from build123d import *

# Parameters (mm, degrees)
SKETCH1_R           = 2.36
SKETCH1_R_2         = 1.625
BOSS_EXTRUDE1_DEPTH = 4.7625


with BuildPart() as part:
    # Sketch1 → Boss-Extrude1 (new body)
    with BuildSketch(Plane(origin=(0, 0, 0), x_dir=(1, 0, 0), z_dir=(0, 1, 0))):
        with BuildLine():
            Line((0, 6.35), (0, 11.65))
            Line((0, 11.65), (-12, 11.65))
            ThreePointArc((-12, 11.65), (-13.212057455, 11.518461446), (-14.367678703, 11.129970522))
            Line((-14.367678703, 11.129970522), (-27.367678703, 5.129970522))
            ThreePointArc((-27.367678703, 5.129970522), (-30.65, 0), (-27.367678703, -5.129970522))
            Line((-27.367678703, -5.129970522), (-14.367678703, -11.129970522))
            ThreePointArc((-14.367678703, -11.129970522), (-8.954912536, -10.759195555), (-6.35, -6))
            Line((-6.35, -6), (-6.35, 0))
            ThreePointArc((-6.35, 0), (-4.490128061, 4.490128061), (0, 6.35))
        make_face()
        with Locations((-25, 0)):
            Circle(SKETCH1_R, mode=Mode.SUBTRACT)
        with Locations((-12, 6)):
            Circle(SKETCH1_R_2, mode=Mode.SUBTRACT)
        with Locations((-12, -6)):
            Circle(SKETCH1_R_2, mode=Mode.SUBTRACT)
    boss_extrude1 = extrude(amount=BOSS_EXTRUDE1_DEPTH)

    # Mirror1: Boss-Extrude1 across plane
    add(boss_extrude1.mirror(Plane(origin=(0, 4.7625, -6.35), x_dir=(0, 0, 1), z_dir=(-1, 0, 0))))


solid = part.part
Can you work these out from the model? Positions are in its coordinate system, mm. Give positions to 0.01 mm unless a question says otherwise; leave off trailing zeros. Order: outer loops, then holes, each group sorted by start corner. A loop starts at its lowest first (then second) coordinate and runs counter-clockwise, first axis right, second up. Notation, with made-up numbers: M 55.5,55 L 98.5,55 A30 ccw 98.5,80 Z; hole C 12.5,12 d11. An arc over 180 degrees is marked long. One line per question, with ' | ' between items.
Item 1: Suppose I cut it at C-C, the plane x = 11. Write out the boundary of the cut face in (y, z).
Answer block:
outline: M 0,-11.65 L 4.76,-11.65 L 4.76,-7.28 L 0,-7.28 Z; M 0,-4.72 L 4.76,-4.72 L 4.76,4.72 L 0,4.72 Z; M 0,7.28 L 4.76,7.28 L 4.76,11.56 L 0,11.56 Z
Item 2: I'm going to push flat-ended pins straight in: pin 1 Ø1.5 at (x, y) = (20, 3) entering from -Z; pin 2 Ø4 at (x, z) = (12, -6) entering from +Y; pin 3 Ø2.5 at (y, z) = (3, 3) entering from -X; pin 4 Ø1 at (x, y) = (15, 1) entering from +Z. Where does each tip first touch, or does it pass through?
Answer block:
pin 1: stops at z = -8.88 | pin 2: stops at y = 4.76 | pin 3: stops at x = -30.37 | pin 4: stops at z = 11.07
Item 3: We'd pull the mould along X, two halves only. Please class faces 1 (the face through (-13.2, 2.35, -11.52)), 2 (the face through (13.2, 2.35, -11.52)), 3 (the face through (-13.623, 2.348, -6.071)): released by +X, released by -X, zero draft, split by the parting line, or undercut.
Answer block:
face 1: released by -X | face 2: released by +X | face 3: undercut
Item 4: Suppose I cut it at D-D, the plane z = 9. Write out the boundary of the cut face in (x, y), then the cut area to 3 significant figures.
Answer block:
outline: M -18.98,0 L -7.21,0 L -7.21,4.76 L -18.98,4.76 Z; M 7.21,0 L 18.98,0 L 18.98,4.76 L 7.21,4.76 Z | area: 112 mm2
Item 5: Please list where these lines run through material, in increasing order: L1, parallel to Z at x = 12, y = 2.7 (3 decimals); L2, parallel to X at y = 3.85, z = 0.
Answer block:
L1: z = -11.65 to -7.625, -4.375 to 4.375, 7.625 to 11.65 | L2: x = -30.65 to -27.36, -22.64 to -6.35, 6.35 to 22.64, 27.36 to 30.65
Item 6: Suppose I cut it at B-B, the plane z = 0.75. Write out the boundary of the cut face in (x, y), then the cut area to 3 significant figures.
Answer block:
outline: M -30.6,0 L -27.24,0 L -27.24,4.76 L -30.6,4.76 Z; M -22.76,0 L -6.35,0 L -6.35,4.76 L -22.76,4.76 Z; M 6.35,0 L 22.76,0 L 22.76,4.76 L 6.35,4.76 Z; M 27.24,0 L 30.6,0 L 30.6,4.76 L 27.24,4.76 Z | area: 188 mm2
Item 7: Suppose I cut it at A-A, the plane y = 4.15. Write out the boundary of the cut face in (x, z) (3 decimals).
Answer block:
outline: M -27.368,-5.13 L -14.368,-11.13 A5.65 ccw -12,-11.65 L 12,-11.65 A5.65 ccw 14.368,-11.13 L 27.368,-5.13 A5.65 ccw 27.368,5.13 L 14.368,11.13 A5.65 ccw 6.35,6 L 6.35,0 A6.35 cw -6.35,0 L -6.35,6 A5.65 ccw -14.368,11.13 L -27.368,5.13 A5.65 ccw Z; hole C -25,0 d4.72; hole C -12,-6 d3.25; hole C -12,6 d3.25; hole C 12,-6 d3.25; hole C 12,6 d3.25; hole C 25,0 d4.72
